Can you work these out from the drawing? Everything is in mm from the part's minimum corner. A direction names the side the tool comes from. Coordinates: 2 decimals unless noted, no trailing zeros. Order: outer loops, then holes, each group sorted by start corner. A loop starts at its lowest first (then second) coordinate and runs counter-clockwise, first axis right, second up. Notation, with made-up numbers: (31, 5) -> (39, 5) arc R14 ccw to (39, 30) -> close; hole circle Ø7 at (24.5, 68.25). An arc over 180 degrees is marked (long way). Return JSON: item names as keys, results as strings. Group by question number.
1) Thinking about a two-plate mould opening in X: for the marked faces 1, 2, 3 and 4, which applies, +X half, -X half, draft (parallel to the pull), parting line (faces both ways), or undercut?
2) If we section it at D-D, the plane y = 50.5: Please give me the cut outline in (x, z) (1 decimal), then the cut area to 3 significant figures.
3) If we section it at B-B, the plane z = 3.75: Please give me the cut outline in (x, y) (1 decimal), then the cut area to 3 significant figures.
4) For the marked faces 5, 6 and 7, which set-ups out of +Z, -Z, +X, -X, +Y, -Y let a thin tool reach every point of the face, with its end or its side?
5) If we section it at C-C, the plane y = 30: Please give me the cut outline in (x, z) (1 decimal).
6) If I drill on probe 1 along X at (y, z) = (13, 6.25) (1 decimal); probe 2 along X at (y, z) = (49, 15.5); probe 3 along Y at (x, z) = (20, 11.25) (1 decimal), over which ranges is the centre line in solid material (lowest first)? Write a range as from..to.
7) If we section it at A-A, the plane y = 21.5: Please give me the cut outline in (x, z) (1 decimal).
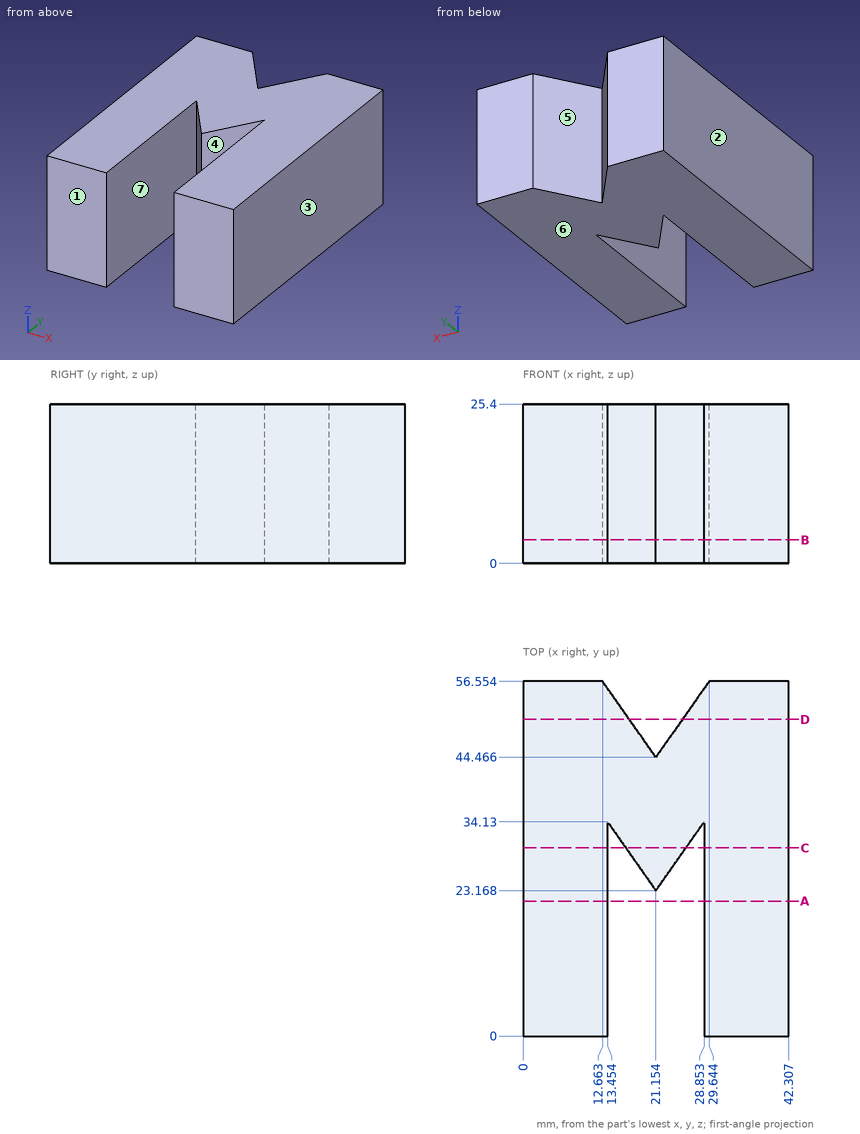
Result sheet:
{
 "1": {"face 1": "draft", "face 2": "-X half", "face 3": "+X half", "face 4": "undercut"},
 "2": {"outline": "(0, 0) -> (16.9, 0) -> (16.9, 25.4) -> (0, 25.4) -> close; (25.4, 0) -> (42.3, 0) -> (42.3, 25.4) -> (25.4, 25.4) -> close", "area": "859 mm2"},
 "3": {"outline": "(0, 0) -> (13.5, 0) -> (13.5, 34.1) -> (21.2, 23.2) -> (28.9, 34.1) -> (28.9, 0) -> (42.3, 0) -> (42.3, 56.6) -> (29.6, 56.6) -> (21.2, 44.5) -> (12.7, 56.6) -> (0, 56.6) -> close", "area": "1,850 mm2"},
 "4": {"face 5": "+Z, -Z, +Y", "face 6": "-Z, +X, -X, +Y, -Y", "face 7": "+Z, -Z, -Y"},
 "5": {"outline": "(0, 0) -> (13.5, 0) -> (13.5, 25.4) -> (0, 25.4) -> close; (16.4, 0) -> (26, 0) -> (26, 25.4) -> (16.4, 25.4) -> close; (28.9, 0) -> (42.3, 0) -> (42.3, 25.4) -> (28.9, 25.4) -> close"},
 "6": {"probe 1": "x = 0..13.5, 28.9..42.3", "probe 2": "x = 0..17.97, 24.34..42.31", "probe 3": "y = 24.8..46.1"},
 "7": {"outline": "(0, 0) -> (13.5, 0) -> (13.5, 25.4) -> (0, 25.4) -> close; (28.9, 0) -> (42.3, 0) -> (42.3, 25.4) -> (28.9, 25.4) -> close"}
}
